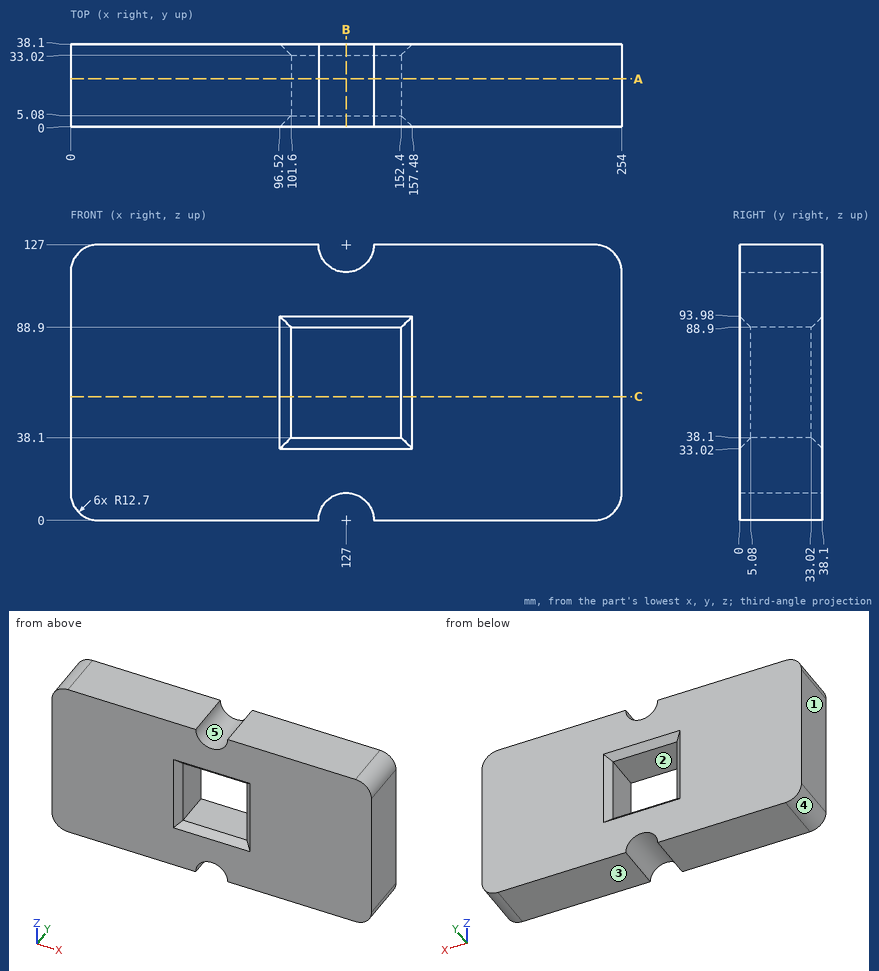
The drawing under review shows one solid part. Ordinate dimensions are in mm from its lowest x, y, z. A direction names the side the tool comes from. Coordinates: 2 decimals unless noted, no trailing zeros. Loops run counter-clockwise (first coordinate to the right, second up) from the corner with the lowest first, then second, coordinate; pieces in that order, holes last. Notation, with made-up numbers: (-14.5, 32) -> (23.5, 32) arc R30 cw to (23.5, 63) -> close; hole circle Ø7 at (15, 65). An arc over 180 degrees is marked (long way). Answer as a JSON object with one key per item and string values.
Q1. Take a section at A-A on y = 22. Give the boundary of the cut face in (x, z).
Answer block:
{"outline": "(0, 12.7) arc R12.7 ccw to (12.7, 0) -> (114.3, 0) arc R12.7 cw to (139.7, 0) -> (241.3, 0) arc R12.7 ccw to (254, 12.7) -> (254, 114.3) arc R12.7 ccw to (241.3, 127) -> (139.7, 127) arc R12.7 cw to (114.3, 127) -> (12.7, 127) arc R12.7 ccw to (0, 114.3) -> close; hole (101.6, 38.1) -> (152.4, 38.1) -> (152.4, 88.9) -> (101.6, 88.9) -> close"}
Q2. Clearance check with flat-ended pins moving along their axes: pin 1 Ø14 at (x, y) = (123.5, 12.5) entering from +Z; pin 2 Ø8.5 at (x, y) = (125, 14) entering from -Z. State where each tip first meets the part, or that it passes through.
Answer block:
{"pin 1": "stops at z = 119.86", "pin 2": "stops at z = 11.06"}
Q3. The part is to be moulded in two halves that separate along X. For the marked faces 3, 4 and 5, say which applies: +X half, -X half, draft (parallel to the pull), parting line (faces both ways), or undercut.
Answer block:
{"face 3": "draft", "face 4": "-X half", "face 5": "undercut"}
Q4. Take a section at B-B on x = 127. Give the boundary of the cut face in (y, z), plus the area to 3 significant figures.
Answer block:
{"outline": "(0, 12.7) -> (38.1, 12.7) -> (38.1, 33.02) -> (33.02, 38.1) -> (5.08, 38.1) -> (0, 33.02) -> close; (0, 93.98) -> (5.08, 88.9) -> (33.02, 88.9) -> (38.1, 93.98) -> (38.1, 114.3) -> (0, 114.3) -> close", "area": "1,880 mm^2"}
Q5. Take a section at C-C on z = 57. Give the boundary of the cut face in (x, y).
Answer block:
{"outline": "(0, 0) -> (96.52, 0) -> (101.6, 5.08) -> (101.6, 33.02) -> (96.52, 38.1) -> (0, 38.1) -> close; (152.4, 5.08) -> (157.48, 0) -> (254, 0) -> (254, 38.1) -> (157.48, 38.1) -> (152.4, 33.02) -> close"}
Q6. Tool access review of the marked faces 1 and 2: name each direction out of +Z, -Z, +X, -X, +Y, -Y from which nothing blocks a thin tool from reaching the whole face with its end or side.
Answer block:
{"face 1": "+Z, -Z, -X, +Y, -Y", "face 2": "+Y, -Y"}
Q7. To check wall thickness, follow L1, parallel to X at y = 29, z = 50; L2, parallel to Z at x = 114, y = 8; L3, parallel to X at y = 3, z = 57. State the ranges of each line that lie inside material, in increasing order.
Answer block:
{"L1": "x = 0 to 101.6, 152.4 to 254", "L2": "z = 0 to 38.1, 88.9 to 127", "L3": "x = 0 to 99.52, 154.48 to 254"}
